Source: CAD feature listing. Evaluate the final solid. Frame: model axes, mm. Face numbers are marked on the shaded views. A direction names the side the tool comes from. Give positions to 0.01 mm unless a question says otherwise; leave off trailing zeros. Order: outer loops, then holes, each group sorted by start corner. A loop starts at its lowest first (then second) coordinate and runs counter-clockwise, first axis right, second up. Notation, with made-up numbers: (-20.75, -7.5) - (-12.75, -7.5) arc R28 cw to (-12.75, 14.5) - close; hole circle Ø1 at (3.25, 28). An arc over 180 degrees is marked (long way). Answer as CSV lines item,"result".
```python
from build123d import *

# Parameters (mm, degrees)
CROQUIS3_W              = 350
CROQUIS3_H              = 450
SALIENTE_EXTRUIR1_DEPTH = 200
VACIADO2_T              = -0.76


with BuildPart() as part:
    # Croquis1 → Recubrir1 section 0
    with BuildSketch(Plane(origin=(0, 0, 0), x_dir=(1, 0, 0), z_dir=(0, 1, 0))):
        with BuildLine():
            Line((-175, 225), (175, 225))
            Line((175, 225), (175, -225))
            Line((175, -225), (-175, -225))
            Line((-175, -225), (-175, 225))
        make_face()
    # Croquis2 → Recubrir1 section 1
    with BuildSketch(Plane(origin=(0, -281.458, 0), x_dir=(1, 0, 0), z_dir=(0, 1, 0))):
        with BuildLine():
            Line((-12.5, 225), (12.5, 225))
            Line((12.5, 225), (12.5, -225))
            Line((12.5, -225), (-12.5, -225))
            Line((-12.5, -225), (-12.5, 225))
        make_face()
    loft()

    # Croquis3 → Saliente-Extruir1 (add)
    with BuildSketch(Plane(origin=(0, 0, 0), x_dir=(1, 0, 0), z_dir=(0, 1, 0))):
        Rectangle(CROQUIS3_W, CROQUIS3_H)
    extrude(amount=SALIENTE_EXTRUIR1_DEPTH)

    # Vaciado2
    vaciado2_openings = [part.faces().sort_by_distance(p)[0] for p in [
        (0, -281.458, 0),
        (0, 200, 0),
    ]]
    offset(amount=VACIADO2_T, openings=vaciado2_openings, kind=Kind.INTERSECTION)


solid = part.part
```
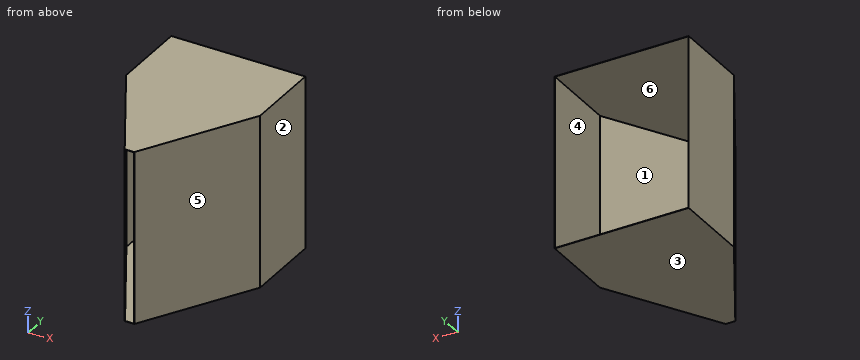
(1) Access query for the marked faces 5 and 6. Directions: +Z, -Z, +X, -X, +Y, -Y. A direction counts if a zero-diameter tool reaches every point of the face in a straight line with its end or side. Return the directions, or none.
Completed:
face 5,"+Z, -Z, +X, -Y"
face 6,"+Y"
(2) Ray query, line 1 (Z direction, x = 30.5, y = 24.5); line 2 (X direction, y = 24, z = 74); line 3 (X direction, y = -162, z = 81). Return the intervals inside material, ascending. Write a range as from..to.
Completed:
line 1,"-225..-224.24, 224.24..225"
line 2,"-175..-174.24, 174.24..175"
line 3,"-81.47..-80.59, 80.59..81.47"
(3) Cut plane D-D (y = -106.5). Return loops of the section in (x, z).
Completed:
outline,"(-113.51, -225) - (113.51, -225) - (113.51, 225) - (-113.51, 225) - close; hole (-112.63, -224.24) - (112.63, -224.24) - (112.63, 224.24) - (-112.63, 224.24) - close"
(4) Cut plane C-C (x = 134.5). Return loops of the section in (y, z).
Completed:
outline,"(-70.15, -225) - (200, -225) - (200, -224.24) - (-68.63, -224.24) - (-68.63, 224.24) - (200, 224.24) - (200, 225) - (-70.15, 225) - close"
(5) Contact query for flat-ended pins moving along their axis: pin 1 (6 mm diameter, centred on y = -142, z = -67, fed in from -X); pin 2 (1.5 mm diameter, centred on y = -9, z = 166, fed in from -X); pin 3 (8 mm diameter, centred on y = -86.5, z = -148, fed in from +X). Output: stop coordinate, or through.
Completed:
pin 1,"x = -94.75"
pin 2,"x = -170.24"
pin 3,"x = 127.37"
(6) Cut plane A-A (z = -77). Return loops of the section in (x, y).
Completed:
outline,"(-175, 0) - (-12.5, -281.46) - (-11.62, -281.46) - (-174.24, 0.2) - (-174.24, 200) - (-175, 200) - close; (11.62, -281.46) - (12.5, -281.46) - (175, 0) - (175, 200) - (174.24, 200) - (174.24, 0.2) - close"
(7) Cut plane B-B (y = 143.5). Return loops of the section in (x, z).
Completed:
outline,"(-175, -225) - (175, -225) - (175, 225) - (-175, 225) - close; hole (-174.24, -224.24) - (174.24, -224.24) - (174.24, 224.24) - (-174.24, 224.24) - close"
(8) Mould query, pull axis X, two halves, no side actions, for the marked faces 1, 2, 3 and 4. Classes: released by +X, released by -X, zero draft, split by the parting line, or undercut.
Completed:
face 1,"undercut"
face 2,"released by +X"
face 3,"zero draft"
face 4,"undercut"
